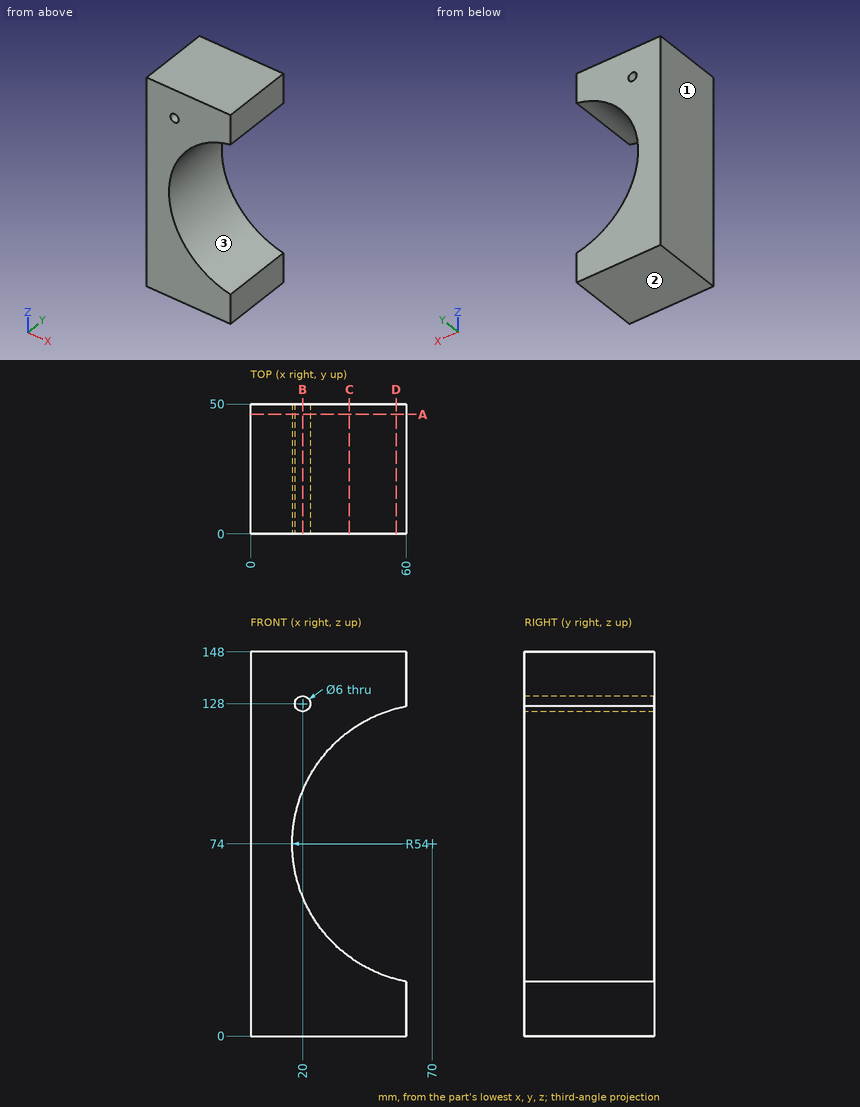
The drawing under review shows one solid part. Ordinate dimensions are in mm from its lowest x, y, z. Coordinates: 2 decimals unless noted, no trailing zeros. Order: outer loops, then holes, each group sorted by start corner. A loop starts at its lowest first (then second) coordinate and runs counter-clockwise, first axis right, second up. Notation, with made-up numbers: (-28.75, 4) -> (-13.75, 4) arc R21 ccw to (-13.75, 26) -> close; hole circle Ø3 at (-14, 22). An arc over 180 degrees is marked (long way). Answer as CSV lines item,"result".
Q1. Wall thickness on line 1 along X through (y, z) = (22, 128); line 2 along Z through (x, y) = (56, 39); line 3 along Z through (x, y) = (27.5, 24): over which ranges is each line inside the solid? List them lowest first. Write a range as [from, to].
Model answer:
line 1,"x = [0, 17], [23, 60]"
line 2,"z = [0, 21.85], [126.15, 148]"
line 3,"z = [0, 40.69], [107.31, 148]"
Q2. We need section D-D (x = 56). State the section outline as (y, z) points, plus the area to 3 significant figures.
Model answer:
outline,"(0, 0) -> (50, 0) -> (50, 21.85) -> (0, 21.85) -> close; (0, 126.15) -> (50, 126.15) -> (50, 148) -> (0, 148) -> close"
area,"2,180 mm2"
Q3. We need section A-A (y = 46). State the section outline as (x, z) points.
Model answer:
outline,"(0, 0) -> (60, 0) -> (60, 20.93) arc R54 cw to (60, 127.07) -> (60, 148) -> (0, 148) -> close; hole circle Ø6 at (20, 128)"
Q4. We need section C-C (x = 38). State the section outline as (y, z) points.
Model answer:
outline,"(0, 0) -> (50, 0) -> (50, 30.5) -> (0, 30.5) -> close; (0, 117.5) -> (50, 117.5) -> (50, 148) -> (0, 148) -> close"
Q5. We need section B-B (x = 20). State the section outline as (y, z) points, plus the area to 3 significant figures.
Model answer:
outline,"(0, 0) -> (50, 0) -> (50, 53.6) -> (0, 53.6) -> close; (0, 94.4) -> (50, 94.4) -> (50, 125) -> (0, 125) -> close; (0, 131) -> (50, 131) -> (50, 148) -> (0, 148) -> close"
area,"5,060 mm2"
Q6. Draft analysis for pull direction Z (two halves, no side actions). For the marked faces 1, 2 and 3, state which applies: released by +Z, released by -Z, zero draft, split by the parting line, or undercut.
Model answer:
face 1,"zero draft"
face 2,"released by -Z"
face 3,"undercut"
